For this review, take the finished solid that the model builds, in its own axes (mm). A direction names the side the tool comes from. Coordinates: 2 decimals unless noted, no trailing zeros. Write each loop counter-clockwise with the first axis right and the second up, starting at its lowest first coordinate (ties: lowest second). Pieces come first, ordered by that corner, then holes. Notation, with made-up numbers: (89, 52.5) - (141, 52.5) arc R30 ccw to (141, 84.5) - close; hole circle Ø7 at (-4.75, 3). An arc over 180 degrees is marked (long way). Use one line per item in the form item = value. Start each with the question number.
1) We need section B-B (x = 8). Give the boundary of the cut face in (y, z), plus the area to 3 significant figures.
2) We need section C-C (z = 1). Give the boundary of the cut face in (x, y) (3 decimals).
3) Tool access review of faces 5 (the flat face through (0, -11, 0)), 6 (the cylindrical face through (0, -9, 8)), 7 (the flat face through (-3, -11.938, 9)), 8 (the flat face through (-3.302, -11, 6)): name each direction out of +Z, -Z, +X, -X, +Y, -Y from which nothing blocks a thin tool from reaching the whole face with its end or side.
4) Mouldability with a two-part tool opening along X and no side actions: class faces 1 (the flat face through (-1.67, -10.69, 3.5)), 2 (the cylindrical face through (3, 18, 4)), 3 (the flat face through (0, -11, 12.7)), 4 (the cylindrical face through (-3.992, -17.977, 6.261)) as pulls with the +X half, pulls with the -X half, needs draft (parallel to the pull), parting line crosses it, or undercut.
5) We need section A-A (y = 0). Give the boundary of the cut face in (x, z) (3 decimals).
6) For L1, parallel to Z at x = 0, y = -8.9; L2, parallel to Y at x = -9.5, z = 1; L3, parallel to Y at x = 10, z = 2.25, list the stretches that pass through material, from the lowest coordinate up. Write a range as from..to.
7) Insertion check: P1, Ø7.5, axis at x = -1, z = 7.5, coming from the -Y side (3 decimals); P2, Ø3, axis at y = -10.5, z = 6, coming from the -X side; P3, Ø2, axis at x = 0, z = 6.35, coming from the +Y side. Each pin has a flat end and moves straight along its axis. Give the tip position at first contact, or say it passes through.
8) We need section D-D (y = -11). Give the boundary of the cut face in (x, z), plus the area to 3 significant figures.
```python
from build123d import *

# Parameters (mm, degrees)
F0_R     = 18.415
F1_DEPTH = 12.7
F2_R     = 1.651
F3_DEPTH = 3.81
F5_DEPTH = 2.54
F6_R     = 3.81
F7_DEPTH = 26.544


with BuildPart() as f1:
    # F0 (on Top) → F1 (new body)
    with BuildSketch(Plane.XY):
        Circle(F0_R)
        with BuildLine():
            ThreePointArc((12.3059, -11.938), (0, -17.145), (-12.3059, -11.938))
            Line((-12.3059, -11.938), (12.3059, -11.938))
        make_face(mode=Mode.SUBTRACT)
        with BuildLine():
            Line((15.095915, -8.128), (-15.095915, -8.128))
            ThreePointArc((-15.095915, -8.128), (0, 17.145), (15.095915, -8.128))
        make_face(mode=Mode.SUBTRACT)
    extrude(amount=F1_DEPTH)

    # F2 (on face) → F3 (cut, through all)
    with BuildSketch(Plane(origin=(0, -8.128, 0), x_dir=(-1, 0, 0), z_dir=(0, 1, 0))):
        with Locations((0, 6.35)):
            Circle(F2_R)
    extrude(amount=-F3_DEPTH, mode=Mode.SUBTRACT)

    # F4 (on face) → F5 (cut)
    with BuildSketch(Plane.XZ.offset(11.938)):
        Polygon((3.302, 4.443589), (3.302, 8.256411), (0, 10.162821), (-3.302, 8.256411), (-3.302, 4.443589), (0, 2.537179), align=None)
    extrude(amount=-F5_DEPTH, mode=Mode.SUBTRACT)

    # F6 (on face) → F7 (cut, through all)
    with BuildSketch(Plane(origin=(0, -8.128, 0), x_dir=(-1, 0, 0), z_dir=(0, 1, 0))):
        with Locations((0, 6.35)):
            Circle(F6_R)
    extrude(amount=F7_DEPTH, mode=Mode.SUBTRACT)


solid = f1.part
```
Determined:
q1.outline = (-16.59, 0) - (-15.16, 0) - (-15.16, 12.7) - (-16.59, 12.7) - close; (-11.94, 0) - (-8.13, 0) - (-8.13, 12.7) - (-11.94, 12.7) - close; (15.16, 0) - (16.59, 0) - (16.59, 12.7) - (15.16, 12.7) - close
q1.area = 84.5 mm²
q2.outline = circle Ø36.83 at (0, 0); hole (-15.096, -8.128) - (15.096, -8.128) arc R17.145 ccw (long way) to start; hole (-12.306, -11.938) arc R17.145 ccw to (12.306, -11.938) - close
q3.face_5 = -Z, +X, -X, +Y, -Y
q3.face_6 = +Y
q3.face_7 = +Z, -Z
q3.face_8 = none
q4.face_1 = undercut
q4.face_2 = undercut
q4.face_3 = needs draft
q4.face_4 = parting line crosses it
q5.outline = (-18.415, 0) - (-17.145, 0) - (-17.145, 12.7) - (-18.415, 12.7) - close; (17.145, 0) - (18.415, 0) - (18.415, 12.7) - (17.145, 12.7) - close
q6.L1 = 0..4.7, 8..12.7
q6.L2 = -15.78..-14.27, -11.94..-8.13, 14.27..15.78
q6.L3 = -15.46..-13.93, -11.94..-8.13, 13.93..15.46
q7.P1 = -18.415
q7.P2 = -16.07
q7.P3 = -17.12
q8.outline = (-14.77, 0) - (14.77, 0) - (14.77, 12.7) - (-14.77, 12.7) - close; hole (-3.3, 4.44) - (0, 2.54) - (3.3, 4.44) - (3.3, 8.26) - (0, 10.16) - (-3.3, 8.26) - close
q8.area = 337 mm²
